Verification items for this drawing (mm, ordinates from the low corner). Give positions to 0.01 mm unless a question says otherwise; leave off trailing zeros. Loops run counter-clockwise (first coordinate to the right, second up) from the corner with the lowest first, then second, coordinate; pieces in that order, holes last. Notation, with made-up numbers: (-30.75, 22.25) -> (-13.75, 22.25) arc R18 cw to (-13.75, 27.25) -> close; hole circle Ø1 at (18.25, -27.5). An arc over 180 degrees is marked (long way). Answer in a Markdown table with one row per item. Add a question column.
Q1. Gauge pin test, flat ends, axial feed: P1, Ø1.5, axis at x = 88.5, y = 8, coming from the -Z side; P2, Ø15, axis at x = 11, y = 31, coming from the -Z side; P3, Ø0.9, axis at y = 39.5, z = 2.5, coming from the -X side. Record the tip position at first contact, or that the pin passes through.
Q2. Section check C-C on x = 79. Enter the section's corners in (y, z) (3 decimals), and give its area (3 significant figures).
Q3. Section check D-D on y = 3.5. Enter the section's corners in (x, z) (3 decimals), and give its area (3 significant figures).
Q4. Section check A-A on x = 95. Enter the section's corners in (y, z).
Q5. Material ranges on probe 1 along Y at (x, z) = (29, 2.35) (3 decimals); probe 2 along X at (y, z) = (8, 4.15); probe 3 along X at (y, z) = (4.5, 1), recorded low to high.
Q6. Section check B-B on y = 24.5. Enter the section's corners in (x, z), and give its area (3 significant figures).
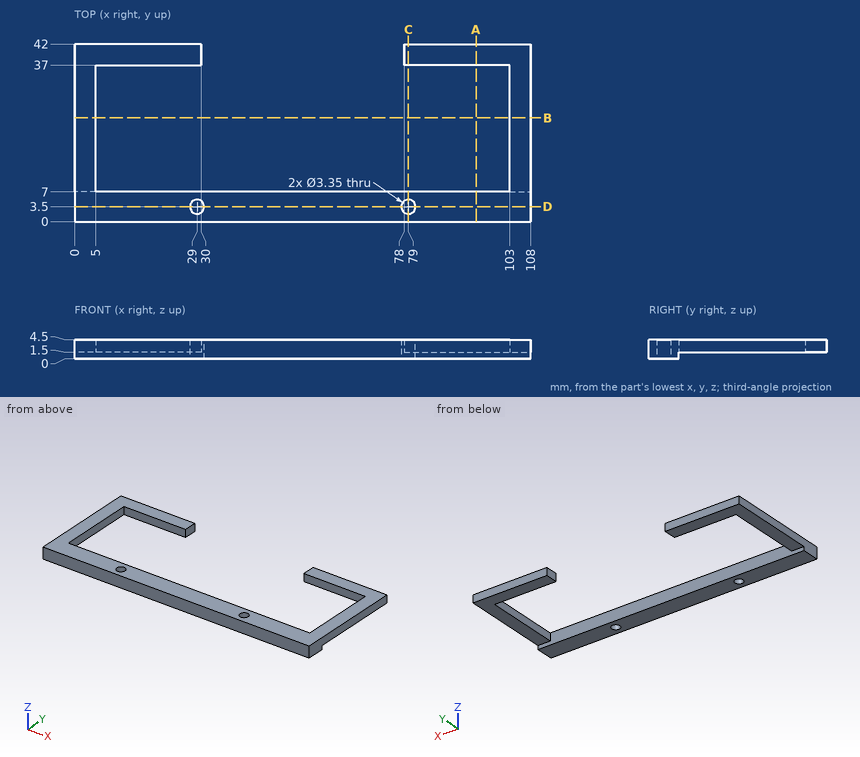
Taken from the geometry:
| question | item | result |
|---|---|---|
| 1 | P1 | passes through |
| 1 | P2 | stops at z = 1.5 |
| 1 | P3 | stops at x = 0 |
| 2 | outline | (0, 0) -> (1.825, 0) -> (1.825, 4.5) -> (0, 4.5) -> close; (5.175, 0) -> (7, 0) -> (7, 4.5) -> (5.175, 4.5) -> close; (37, 1.5) -> (42, 1.5) -> (42, 4.5) -> (37, 4.5) -> close |
| 2 | area | 31.4 mm² |
| 3 | outline | (0, 0) -> (27.325, 0) -> (27.325, 4.5) -> (0, 4.5) -> close; (30.675, 0) -> (77.325, 0) -> (77.325, 4.5) -> (30.675, 4.5) -> close; (80.675, 0) -> (108, 0) -> (108, 4.5) -> (80.675, 4.5) -> close |
| 3 | area | 456 mm² |
| 4 | outline | (0, 0) -> (7, 0) -> (7, 4.5) -> (0, 4.5) -> close; (37, 1.5) -> (42, 1.5) -> (42, 4.5) -> (37, 4.5) -> close |
| 5 | probe 1 | y = 0 to 1.825, 5.175 to 7, 37 to 42 |
| 5 | probe 2 | x = 0 to 5, 103 to 108 |
| 5 | probe 3 | x = 0 to 27.66, 30.34 to 77.66, 80.34 to 108 |
| 6 | outline | (0, 1.5) -> (5, 1.5) -> (5, 4.5) -> (0, 4.5) -> close; (103, 1.5) -> (108, 1.5) -> (108, 4.5) -> (103, 4.5) -> close |
| 6 | area | 30.0 mm² |
